Input: part model. Units: mm. Frame: model coordinates. Face numbers are marked on the shaded views. A direction names the side the tool comes from. Give positions to 0.01 mm unless a question says otherwise; leave off trailing zeros. Loops run counter-clockwise (first coordinate to the right, second up) from the corner with the lowest first, then second, coordinate; pieces in that order, holes last. Notation, with made-up numbers: M 58,38.25 L 75,38.25 A14 ccw 75,56.25 Z; hole C -1,70.25 d1. An arc over 180 degrees is marked long. Answer as a JSON object with one key per item and string values. Group by question number.
1) Access query for the marked faces 1 and 2. Directions: +Z, -Z, +X, -X, +Y, -Y. A direction counts if a zero-diameter tool reaches every point of the face in a straight line with its end or side. Return the directions, or none.
2) Section query B-B on y = -11.5. Return loops of the section in (x, z), plus the area to 3 significant figures.
3) Ray query, L1, parallel to Y at x = 55, z = 4; L2, parallel to Z at x = 12.7, y = -15.5; L3, parallel to Y at x = 60, z = 12. Return the intervals inside material, ascending.
4) First-contact query: P1, Ø3, axis at x = 37.5, y = -16, coming from the -Z side; P2, Ø7.5, axis at x = 38, y = -17.5, coming from the +Z side; P3, Ø5, axis at x = 7.5, y = -13.5, coming from the +Z side. Flat tips, straight axial feed; report the tip coordinate or a pass-through.
5) Draft query along X for the marked faces 3, 4 and 5. Return one class per face: +X half, -X half, draft (parallel to the pull), parting line (faces both ways), or undercut.
6) Section query C-C on z = 7. Return loops of the section in (x, y), plus the area to 3 significant figures.
7) Section query D-D on x = 45.5. Return loops of the section in (y, z).
8) Section query A-A on z = 24.5. Return loops of the section in (x, y).
from build123d import *

# Parameters (mm, degrees)
F1_DEPTH = 25.4
F2_R     = 6.35
F3_DEPTH = 25.4
F4_DEPTH = 25.4
F7_DEPTH = 12.7


with BuildPart() as f1:
    # F0 (on Front) → F1 (new body)
    with BuildSketch(Plane.XZ):
        Polygon((25.4, 38.1), (0, 38.1), (0, 0), (69.85, 0), (69.85, 12.7), (25.4, 12.7), align=None)
    extrude(amount=F1_DEPTH)

    # F2 (on face) → F3 (cut)
    with BuildSketch(Plane.XZ.offset(25.4)):
        with Locations((12.7, 25.4)):
            Circle(F2_R)
    extrude(amount=-F3_DEPTH, mode=Mode.SUBTRACT)

    # F2 (on face) → F4 (cut)
    with BuildSketch(Plane.XZ.offset(25.4)):
        with BuildLine():
            ThreePointArc((0, 25.4), (3.719744, 34.380256), (12.7, 38.1))
            Line((12.7, 38.1), (0, 38.1))
            Line((0, 38.1), (0, 25.4))
        make_face()
        with BuildLine():
            ThreePointArc((12.7, 38.1), (21.680256, 34.380256), (25.4, 25.4))
            Line((25.4, 25.4), (25.4, 38.1))
            Line((25.4, 38.1), (12.7, 38.1))
        make_face()
    extrude(amount=-F4_DEPTH, mode=Mode.SUBTRACT)

    # F6 (on face) → F7 (cut)
    with BuildSketch(Plane.XY.offset(12.7)):
        with BuildLine():
            ThreePointArc((38.260814, -19.047963), (42.646629, -17.132907), (44.45, -12.7))
            ThreePointArc((44.45, -12.7), (42.64191, -8.262258), (38.247307, -6.351709))
            ThreePointArc((38.247307, -6.351709), (31.751886, -12.545255), (37.937817, -19.047929))
            Line((37.937817, -19.047929), (38.260814, -19.047963))
        make_face()
        with BuildLine():
            ThreePointArc((38.247307, -6.351709), (42.64191, -8.262258), (44.45, -12.7))
            ThreePointArc((44.45, -12.7), (42.646629, -17.132907), (38.260814, -19.047963))
            Line((38.260814, -19.047963), (57.149315, -19.05))
            ThreePointArc((57.149315, -19.05), (50.8, -12.699945), (57.149426, -6.35))
            Line((57.149426, -6.35), (38.247307, -6.351709))
        make_face()
        with BuildLine():
            ThreePointArc((37.937817, -19.047929), (38.099315, -19.05), (38.260814, -19.047963))
            Line((38.260814, -19.047963), (37.937817, -19.047929))
        make_face()
        with BuildLine():
            ThreePointArc((63.5, -12.7), (61.639925, -8.209669), (57.149426, -6.35))
            ThreePointArc((57.149426, -6.35), (50.8, -12.699945), (57.149315, -19.05))
            ThreePointArc((57.149315, -19.05), (61.639886, -17.19037), (63.5, -12.7))
        make_face()
    extrude(amount=-F7_DEPTH, mode=Mode.SUBTRACT)


solid = f1.part
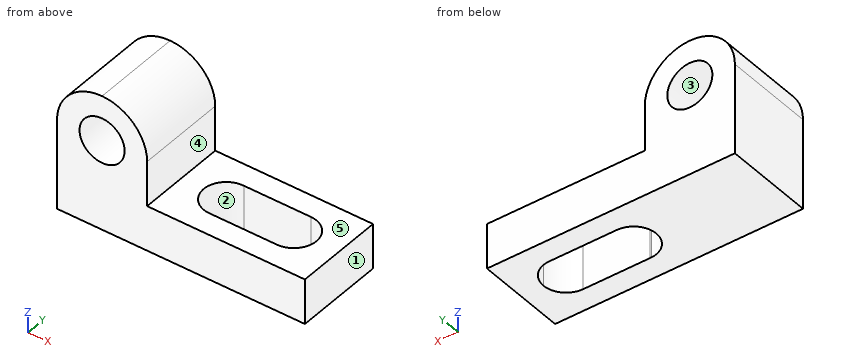
Output:
{
 "1": {"face 1": "+Z, -Z, +X, +Y, -Y", "face 2": "+Z, -Z"},
 "2": {"outline": "M 0,0 L 31.86,0 L 31.86,12.7 L 25.4,12.7 L 25.4,25.4 A12.7 ccw 0,25.4 Z; M 63.39,0 L 69.85,0 L 69.85,12.7 L 63.39,12.7 Z; hole C 12.7,25.4 d12.7", "area": "936 mm^2"},
 "3": {"L1": "y = -25.4 to -19.05, -6.35 to 0", "L2": "z = 0 to 19.05, 31.75 to 38.1", "L3": "y = -25.4 to -18.37, -7.03 to 0"},
 "4": {"P1": "passes through", "P2": "stops at z = 12.7", "P3": "stops at z = 37.81"},
 "5": {"face 3": "undercut", "face 4": "+X half", "face 5": "draft"},
 "6": {"outline": "M 0,-25.4 L 69.85,-25.4 L 69.85,0 L 0,0 Z; hole M 37.94,-19.05 A6.35 ccw 38.26,-19.05 L 57.15,-19.05 A6.35 ccw 57.15,-6.35 L 38.25,-6.35 A6.35 ccw Z", "area": "1,410 mm^2"},
 "7": {"outline": "M -25.4,0 L -19.05,0 L -19.05,12.7 L -25.4,12.7 Z; M -6.35,0 L 0,0 L 0,12.7 L -6.35,12.7 Z"},
 "8": {"outline": "M 0,-25.4 L 6.41,-25.4 L 6.41,0 L 0,0 Z; M 18.99,-25.4 L 25.4,-25.4 L 25.4,0 L 18.99,0 Z"}
}
